Check sheet for the modelled part. Datum: model origin and axes. Units: mm. Face numbers are marked on the shaded views. Round coordinates to 2 decimals unless told otherwise and drop trailing zeros. Write each loop counter-clockwise with the first axis right and the second up, starting at its lowest first coordinate (ties: lowest second). Pieces come first, ordered by that corner, then holes. Notation, with made-up numbers: (53.25, 49) - (90.25, 49) arc R10 cw to (90.25, 66) - close; hole circle Ø8 at (-27, -24). An arc over 180 degrees is marked (long way). Use one line per item in the form item = value. Start each with the question number.
1) Scan lines: probe 1 along X at (y, z) = (-40.5, 66); probe 2 along X at (y, z) = (-31, 81.5); probe 3 along Y at (x, z) = (449, 51.5). Record each from-to range of solid material in increasing order.
2) Section check A-A (y = -43). Record the boundary of the cut face in (x, z).
3) Section check B-B (x = 298.5). Record the boundary of the cut face in (y, z), then the cut area to 3 significant figures.
4) Section check C-C (z = 107.5). Record the boundary of the cut face in (x, y), then the cut area to 3 significant figures.
5) Draft check along X on the marked faces 1, 2 and 3. Enter one of: +X half, -X half, draft (parallel to the pull), parting line (faces both ways), or undercut.
6) Gauge pin test, flat ends, axial feed: P1, Ø4, axis at y = -34, z = 96.5, coming from the -X side; P2, Ø4, axis at y = -21.5, z = 69, coming from the -X side; P3, Ø1, axis at x = 209, z = 67, coming from the -Y side. Record the tip position at first contact, or that the pin passes through.
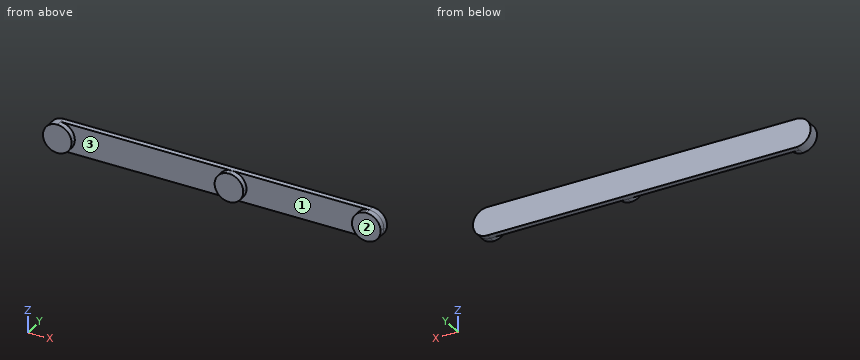
from build123d import *

# Parameters (mm, degrees)
F1_DEPTH = 25.4
F3_DEPTH = 25.4


with BuildPart() as f1:
    # F0 (on Front) → F1 (new body)
    with BuildSketch(Plane.XZ):
        with BuildLine():
            ThreePointArc((0, 127), (-63.5, 63.5), (0, 0))
            Line((0, 0), (1371.6, 0))
            ThreePointArc((1371.6, 0), (1435.1, 63.5), (1371.6, 127))
            Line((1371.6, 127), (0, 127))
        make_face()
    extrude(amount=F1_DEPTH)

    # F2 (on face) → F3 (join)
    with BuildSketch(Plane.XZ.offset(25.4)):
        with BuildLine():
            ThreePointArc((0, 0), (44.901281, 18.598719), (63.5, 63.5))
            ThreePointArc((63.5, 63.5), (44.901281, 108.401281), (0, 127))
            ThreePointArc((0, 127), (-63.5, 63.5), (0, 0))
        make_face()
        with BuildLine():
            ThreePointArc((825.5, 63.5), (806.901281, 108.401281), (762, 127))
            ThreePointArc((762, 127), (698.5, 63.5), (762, 0))
            ThreePointArc((762, 0), (806.901281, 18.598719), (825.5, 63.5))
        make_face()
        with BuildLine():
            ThreePointArc((1435.1, 63.5), (1416.501281, 108.401281), (1371.6, 127))
            ThreePointArc((1371.6, 127), (1308.1, 63.5), (1371.6, 0))
            ThreePointArc((1371.6, 0), (1416.501281, 18.598719), (1435.1, 63.5))
        make_face()
    extrude(amount=F3_DEPTH)


solid = f1.part
Results are:
q1.probe_1 = -63.45 to 63.45, 698.55 to 825.45, 1308.15 to 1435.05
q1.probe_2 = -60.9 to 60.9, 701.1 to 822.9, 1310.7 to 1432.5
q1.probe_3 = -25.4 to 0
q2.outline = (0, 0) arc R63.5 ccw to (63.5, 63.5) arc R63.5 ccw to (0, 127) arc R63.5 ccw to start; (762, 0) arc R63.5 ccw to (825.5, 63.5) arc R63.5 ccw to (762, 127) arc R63.5 ccw to start; (1371.6, 0) arc R63.5 ccw to (1435.1, 63.5) arc R63.5 ccw to (1371.6, 127) arc R63.5 ccw to start
q3.outline = (-25.4, 0) - (0, 0) - (0, 127) - (-25.4, 127) - close
q3.area = 3,230 mm²
q4.outline = (-45.78, -50.8) - (45.78, -50.8) - (45.78, -25.4) - (716.22, -25.4) - (716.22, -50.8) - (807.78, -50.8) - (807.78, -25.4) - (1325.82, -25.4) - (1325.82, -50.8) - (1417.38, -50.8) - (1417.38, 0) - (-45.78, 0) - close
q4.area = 44,100 mm²
q5.face_1 = undercut
q5.face_2 = draft
q5.face_3 = undercut
q6.P1 = -55.42
q6.P2 = -63.4
q6.P3 = -25.4
